Can you work these out from the model? Positions are in its coordinate system, mm. A direction names the side the tool comes from. Round coordinates to 2 decimals unless told otherwise and drop trailing zeros. Loops run counter-clockwise (first coordinate to the right, second up) from the corner with the lowest first, then second, coordinate; pieces in that order, holes last. Notation, with made-up numbers: M 0.25,89 L 21.25,89 A19 ccw 21.25,101 Z; hole C 56.25,34.5 d11. An arc over 180 degrees is marked long. Return JSON: item names as keys, results as strings.
```python
from build123d import *

# Parameters (mm, degrees)
F1_DEPTH = 25.4
F2_W     = 12.7
F2_H     = 31.75
F3_DEPTH = 25.4


with BuildPart() as f1:
    # F0 (on Right) → F1 (new body)
    with BuildSketch(Plane.YZ):
        Polygon((-25.4, 0), (0, 0), (0, 31.75), (-5.158795, 31.75), (-25.4, 6.35), align=None)
    extrude(amount=F1_DEPTH)

    # F2 (on Front) → F3 (join)
    with BuildSketch(Plane.XZ):
        with Locations((-6.35, 15.875)):
            Rectangle(F2_W, F2_H)
    extrude(amount=F3_DEPTH)


solid = f1.part
```
Q1. Suppose I cut it at A-A, the plane x = 2.5. Please give me the cut outline in (y, z).
Results:
{"outline": "M -25.4,0 L 0,0 L 0,31.75 L -5.16,31.75 L -25.4,6.35 Z"}
Q2. On a 3-axis mill with a long thin cutter (end or side, diameter ignored), from which of +Z, -Z, +X, -X, +Y, -Y can I reach the whole of each face in a straight line? I mean faces 1 (the flat face through (0, -20, 25)), 2 (the flat face through (25.4, -10, 13)). Say none if no direction works.
Results:
{"face 1": "+Z, +X, -Y", "face 2": "+Z, -Z, +X, +Y, -Y"}
Q3. I'm going to push flat-ended pins straight in: pin 1 Ø3 at (x, y) = (-6.5, -9) entering from -Z; pin 2 Ø8 at (x, z) = (5, 12) entering from -Y; pin 3 Ø5 at (x, z) = (12, 20) entering from -Y. Where does each tip first touch, or does it pass through?
Results:
{"pin 1": "stops at z = 0", "pin 2": "stops at y = -24.09", "pin 3": "stops at y = -16.51"}
Q4. If I drill on line 1 along X through (y, z) = (-22, 26.5); line 2 along Y through (x, z) = (24.5, 28); line 3 along Y through (x, z) = (9, 14), over which ranges is the centre line in solid material (lowest first)?
Results:
{"line 1": "x = -12.7 to 0", "line 2": "y = -8.15 to 0", "line 3": "y = -19.3 to 0"}
Q5. Suppose I cut it at B-B, the plane z = 8. Please give me the cut outline in (x, y).
Results:
{"outline": "M -12.7,-25.4 L 0,-25.4 L 0,-24.09 L 25.4,-24.09 L 25.4,0 L -12.7,0 Z"}
Q6. Suppose I cut it at C-C, the plane y = -21.5. Please give me the cut outline in (x, z).
Results:
{"outline": "M -12.7,0 L 25.4,0 L 25.4,11.24 L 0,11.24 L 0,31.75 L -12.7,31.75 Z"}
